Part model, mm, in its own coordinate system. A direction names the side the tool comes from. Round coordinates to 2 decimals unless told otherwise and drop trailing zeros. Write each loop counter-clockwise with the first axis right and the second up, starting at its lowest first coordinate (ties: lowest second). Pieces come first, ordered by that corner, then holes. Notation, with made-up numbers: (35, 20.5) -> (67, 20.5) arc R15 ccw to (67, 30.5) -> close; hole circle Ø1 at (-33.75, -8). An arc over 180 degrees is marked (long way). Return JSON: item names as keys, results as strings. Group by question number.
```python
from build123d import *

# Parameters (mm, degrees)
SKETCH1_W           = 91
SKETCH1_H           = 55
BOSS_EXTRUDE1_DEPTH = 90
SKETCH2_W           = 24
SKETCH2_H           = 6
CUT_EXTRUDE1_DEPTH  = 91
SKETCH3_W           = 14
SKETCH3_H           = 17
CUT_EXTRUDE2_DEPTH  = 91


with BuildPart() as part:
    # Sketch1 → Boss-Extrude1 (new body)
    with BuildSketch(Plane.XY):
        with Locations((45.5, 27.5)):
            Rectangle(SKETCH1_W, SKETCH1_H)
    extrude(amount=BOSS_EXTRUDE1_DEPTH)

    # Sketch2 → Cut-Extrude1 (cut, through all)
    with BuildSketch(Plane.XY.offset(90)):
        with Locations((79, 52)):
            Rectangle(SKETCH2_W, SKETCH2_H)
        with Locations((12, 52)):
            Rectangle(SKETCH2_W, SKETCH2_H)
    extrude(amount=-CUT_EXTRUDE1_DEPTH, mode=Mode.SUBTRACT)

    # Sketch3 → Cut-Extrude2 (cut, through all)
    with BuildSketch(Plane.XY.offset(90)):
        with Locations((84, 40.5)):
            Rectangle(SKETCH3_W, SKETCH3_H)
        with Locations((7, 40.5)):
            Rectangle(SKETCH3_W, SKETCH3_H)
    extrude(amount=-CUT_EXTRUDE2_DEPTH, mode=Mode.SUBTRACT)


solid = part.part
```
Item 1: Flat gauge pins, fed straight in: P1, Ø11, axis at x = 18, z = 29.5, coming from the +Y side; P2, Ø3, axis at y = 44, z = 28.5, coming from the -X side; P3, Ø1.8, axis at y = 52.5, z = 37, coming from the -X side. Where does each tip first touch, or does it go through?
Item 2: Cut at A-A (z = 55). Write the cut outline in (x, y).
Item 3: Wall check: L1, parallel to Y at x = 15, z = 70.5; L2, parallel to X at y = 36, z = 28; L3, parallel to Y at x = 13, z = 84.5. Give the ranges that are in metal, low to high.
Item 4: Cut at C-C (x = 81.5). Write the cut outline in (y, z), then the cut area to 3 significant figures.
Item 5: Cut at B-B (y = 45). Write the cut outline in (x, z), then the cut area to 3 significant figures.
Item 6: Which spindle directions (+Z, -Z, +X, -X, +Y, -Y) get a long thin tool onto all of the face, cutting with end or side? Do faces 1 (the face through (14, 40, 46)), 2 (the face through (0, 16, 44)), 3 (the face through (72, 49, 46)). Say none if no direction does.
Checks:
{
 "1": {"P1": "stops at y = 49", "P2": "stops at x = 14", "P3": "stops at x = 24"},
 "2": {"outline": "(0, 0) -> (91, 0) -> (91, 32) -> (77, 32) -> (77, 49) -> (67, 49) -> (67, 55) -> (24, 55) -> (24, 49) -> (14, 49) -> (14, 32) -> (0, 32) -> close"},
 "3": {"L1": "y = 0 to 49", "L2": "x = 14 to 77", "L3": "y = 0 to 32"},
 "4": {"outline": "(0, 0) -> (32, 0) -> (32, 90) -> (0, 90) -> close", "area": "2,880 mm2"},
 "5": {"outline": "(14, 0) -> (77, 0) -> (77, 90) -> (14, 90) -> close", "area": "5,670 mm2"},
 "6": {"face 1": "+Z, -Z, -X, +Y", "face 2": "+Z, -Z, -X, +Y, -Y", "face 3": "+Z, -Z, +X, +Y"}
}
